Build history of the part. All positions in model axes, mm. A direction names the side the tool comes from. Give positions to 0.01 mm unless a question says otherwise; leave off trailing zeros. Write each loop counter-clockwise with the first axis right and the second up, starting at its lowest first coordinate (ties: lowest second). Pieces come first, ordered by that corner, then holes. Notation, with made-up numbers: M 25,45.5 L 63,45.5 A22 ccw 63,60.5 Z; hole C -18.5,47.25 d9. An arc over 180 degrees is marked long. One line per item, written item: value. Start each with the question number.
from build123d import *

# Parameters (mm, degrees)
BOSS_EXTRUDE1_DEPTH     = 38.1
CUT_EXTRUDE1_DEPTH      = 55.4
CUT_EXTRUDE1_DEPTH_BACK = 30
SKETCH2_R               = 4
SKETCH3_R               = 6.5
CUT_EXTRUDE2_DEPTH      = 18.2
CUT_EXTRUDE3_START      = 19
SKETCH4_W               = 24
SKETCH4_H               = 20
CUT_EXTRUDE3_DEPTH      = 10
CHAMFER1_SIZE           = 3


with BuildPart() as part:
    # Sketch1 → Boss-Extrude1 (new body)
    with BuildSketch(Plane.XY):
        with BuildLine():
            Line((-10, -15.714961024), (-10, 14.285038976))
            Line((-10, 14.285038976), (0, 14.285038976))
            Line((0, 14.285038976), (0, 1))
            ThreePointArc((0, 1), (-0.707106781, -0.707106781), (1, 0))
            Line((1, 0), (18, 0))
            Line((18, 0), (18, -3.779961024))
            Line((18, -3.779961024), (23.5, -3.779961024))
            Line((23.5, -3.779961024), (23.5, -11.899961024))
            Line((23.5, -11.899961024), (19, -11.899961024))
            Line((19, -11.899961024), (19, -15.714961024))
            Line((19, -15.714961024), (-10, -15.714961024))
        make_face()
    extrude(amount=-BOSS_EXTRUDE1_DEPTH)

    # Sketch2 → Cut-Extrude1 (cut, two sides: drawn at the far end of the back side and taken through both)
    with BuildSketch(Plane(origin=(0, 0, 0), x_dir=(0, 0, -1), z_dir=(1, 0, 0)).offset(-CUT_EXTRUDE1_DEPTH_BACK)):
        with Locations((-19.05, -7.839961024)):
            Circle(SKETCH2_R)
        with Locations((19.05, -7.839961024)):
            Circle(SKETCH2_R)
    extrude(amount=CUT_EXTRUDE1_DEPTH + CUT_EXTRUDE1_DEPTH_BACK, mode=Mode.SUBTRACT)

    # Sketch3 → Cut-Extrude2 (cut)
    with BuildSketch(Plane(origin=(0, 0, 0), x_dir=(0, 0, -1), z_dir=(1, 0, 0))):
        with Locations((19.05, -7.839961024)):
            Circle(SKETCH3_R)
    extrude(amount=-CUT_EXTRUDE2_DEPTH, mode=Mode.SUBTRACT)

    # Sketch4 → Cut-Extrude3 (cut)
    with BuildSketch(Plane(origin=(0, 0, 0), x_dir=(0, 0, -1), z_dir=(1, 0, 0)).offset(CUT_EXTRUDE3_START)):
        with Locations((19.05, -7.839961024)):
            Rectangle(SKETCH4_W, SKETCH4_H)
    extrude(amount=CUT_EXTRUDE3_DEPTH, mode=Mode.SUBTRACT)

    # Chamfer1
    chamfer1_edges = [part.edges().sort_by_distance(p)[0] for p in [
        (23.5, -3.779961024, -34.575),
        (23.5, -11.899961024, -34.575),
        (23.5, -11.899961024, -3.525),
        (23.5, -3.779961024, -3.525),
    ]]
    chamfer(chamfer1_edges, length=CHAMFER1_SIZE)


solid = part.part
1) Band-saw the part on C-C (y = -6). List the corners of the cut face in (x, z), then the cut area to 3 significant figures.
2) Drop flat-ended pins along their axis: P1, Ø10.5, axis at y = -7.84, z = -19.05, coming from the +X side; P2, Ø2, axis at y = 2, z = -23.5, coming from the +X side; P3, Ø4, axis at y = -6, z = -18.5, coming from the -X side; P4, Ø0.8, axis at x = 19, z = -12, coming from the +Y side. Give the stop position or say it passes through.
3) Band-saw the part on B-B (z = -19.05). List the corners of the cut face in (x, y).
4) Band-saw the part on A-A (x = 20). List the corners of the cut face in (y, z), then the cut area to 3 significant figures.
5) Band-saw the part on D-D (z = -6). List the corners of the cut face in (x, y).
6) Tool access for faces 4 (the face through (20, -11.9, -3)), 5 (the face through (21, -8, -7.05)), 6 (the face through (9, 0, -19)), 7 (the face through (3, -4, -38.1)), 8 (the face through (-4.93, -11.795, -13.892)): list every direction of +Z, -Z, +X, -X, +Y, -Y with a clear straight run to the whole face (end or side of a thin tool).
7) Mould opens along Y. For faces 1 (the face through (23.5, -8, -35)), 2 (the face through (5, -15.715, -19)), 3 (the face through (-0.73, -0.683, -18.783)) say: released by +Y, released by -Y, zero draft, split by the parting line, or undercut.
8) Probe line 1 along Y through (x, z) = (7, -19); line 2 along Y through (x, z) = (-3.25, -19.05); line 3 along X through (y, z) = (10.75, -28.5). List the from-to ranges inside material, lowest first. Write a range as from..to.
Model answer:
1. outline: M -10,-38.1 L 22.72,-38.1 L 22.72,-31.05 L 19,-31.05 L 19,-22.6 L 0,-22.6 L 0,-25.28 L -10,-25.28 Z; M -10,-12.82 L 0,-12.82 L 0,-15.5 L 19,-15.5 L 19,-7.05 L 22.72,-7.05 L 22.72,0 L -10,0 Z
1. area: 898 mm²
2. P1: stops at x = 19
2. P2: stops at x = 0
2. P3: passes through
2. P4: stops at y = -3.78
3. outline: M -10,-15.71 L 19,-15.71 L 19,-11.84 L 0,-11.84 L 0,-14.34 L -10,-14.34 Z; M -10,-1.34 L 0,-1.34 L 0,-3.84 L 19,-3.84 L 19,-3.78 L 18,-3.78 L 18,0 L 1,0 A1 cw long 0,1 L 0,14.29 L -10,14.29 Z
4. outline: M -11.9,-38.1 L -3.78,-38.1 L -3.78,-31.05 L -11.9,-31.05 Z; M -11.9,-7.05 L -3.78,-7.05 L -3.78,0 L -11.9,0 Z
4. area: 114 mm²
5. outline: M -10,-15.71 L 19,-15.71 L 19,-11.9 L 20.5,-11.9 L 23.5,-8.9 L 23.5,-6.78 L 20.5,-3.78 L 18,-3.78 L 18,0 L 1,0 A1 cw long 0,1 L 0,14.29 L -10,14.29 Z
6. face 4: +Z, -Z, +X, -Y
6. face 5: +X, +Y, -Y
6. face 6: +Z, -Z, +X, +Y
6. face 7: -Z, +X, -X, +Y, -Y
6. face 8: -X
7. face 1: zero draft
7. face 2: released by -Y
7. face 3: undercut
8. line 1: y = -15.71..-11.84, -3.84..0
8. line 2: y = -15.71..-14.34, -1.34..14.29
8. line 3: x = -10..0
